The drawing under review shows one solid part. Ordinate dimensions are in mm from its lowest x, y, z. Coordinates: 2 decimals unless noted, no trailing zeros. Answer as a JSON object with one key per item and string values. Group by question number.
1. Consider section A-A (y = 1.25). Count the separate pieces of the cut face and the enclosed holes in it, then the cut area to 3 significant figures.
2. To check wall thickness, follow probe 1 along X at (y, z) = (5, 88.9) (1 decimal); probe 2 along X at (y, z) = (4, 88.9); probe 3 along X at (y, z) = (5.5, 49). State the ranges of each line that lie inside material, in increasing order.
3. Insertion check: pin 1 (1 mm diameter, centred on x = 321.5, y = 5.5, fed in from +Z); pin 2 (3 mm diameter, centred on x = 345, y = 1, fed in from -Z). Each pin has a flat end and moves straight along its axis. Give the tip position at first contact, or say it passes through.
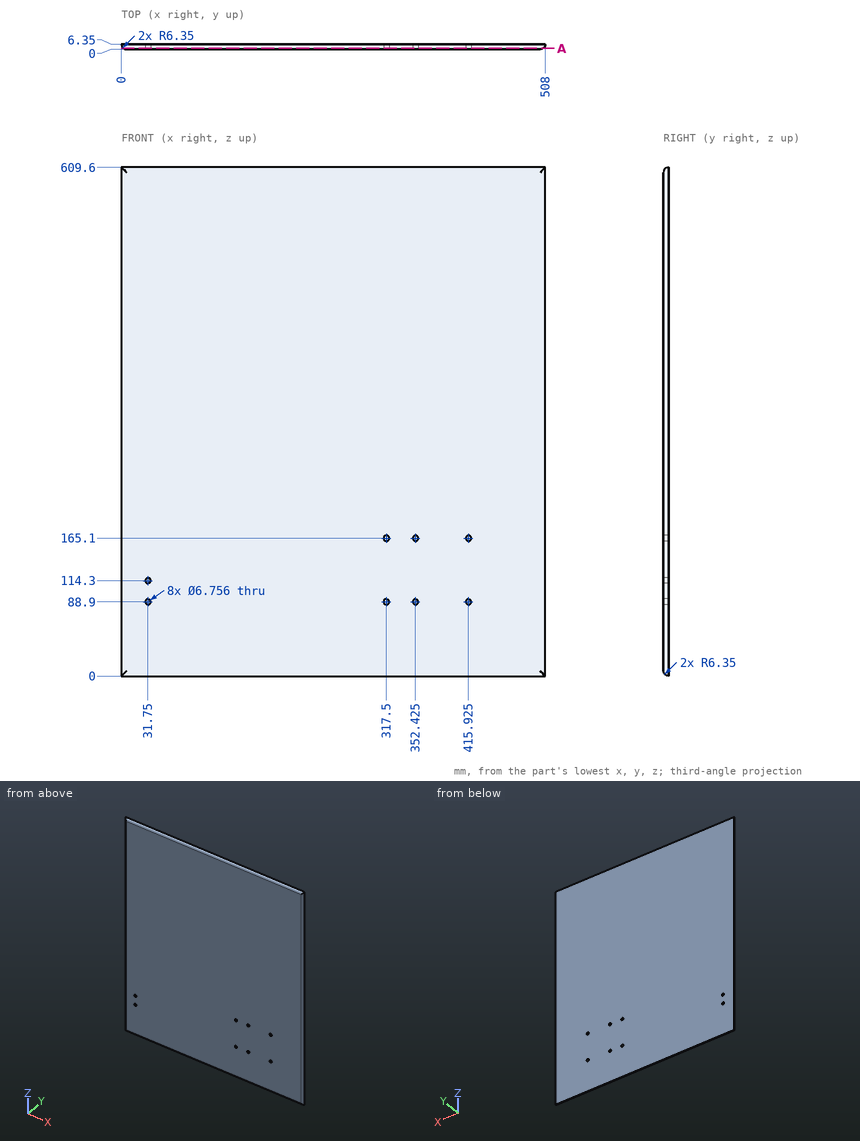
Findings below:
{
 "1": {"separate pieces": "1", "enclosed holes": "8", "area": "304,000 mm^2"},
 "2": {"probe 1": "x = 0.1 to 28.4, 35.1 to 314.1, 320.9 to 349, 355.8 to 412.5, 419.3 to 507.9", "probe 2": "x = 0.45 to 28.37, 35.13 to 314.12, 320.88 to 349.05, 355.8 to 412.55, 419.3 to 507.55", "probe 3": "x = 0.06 to 507.94"},
 "3": {"pin 1": "stops at z = 609.59", "pin 2": "stops at z = 1.3"}
}
